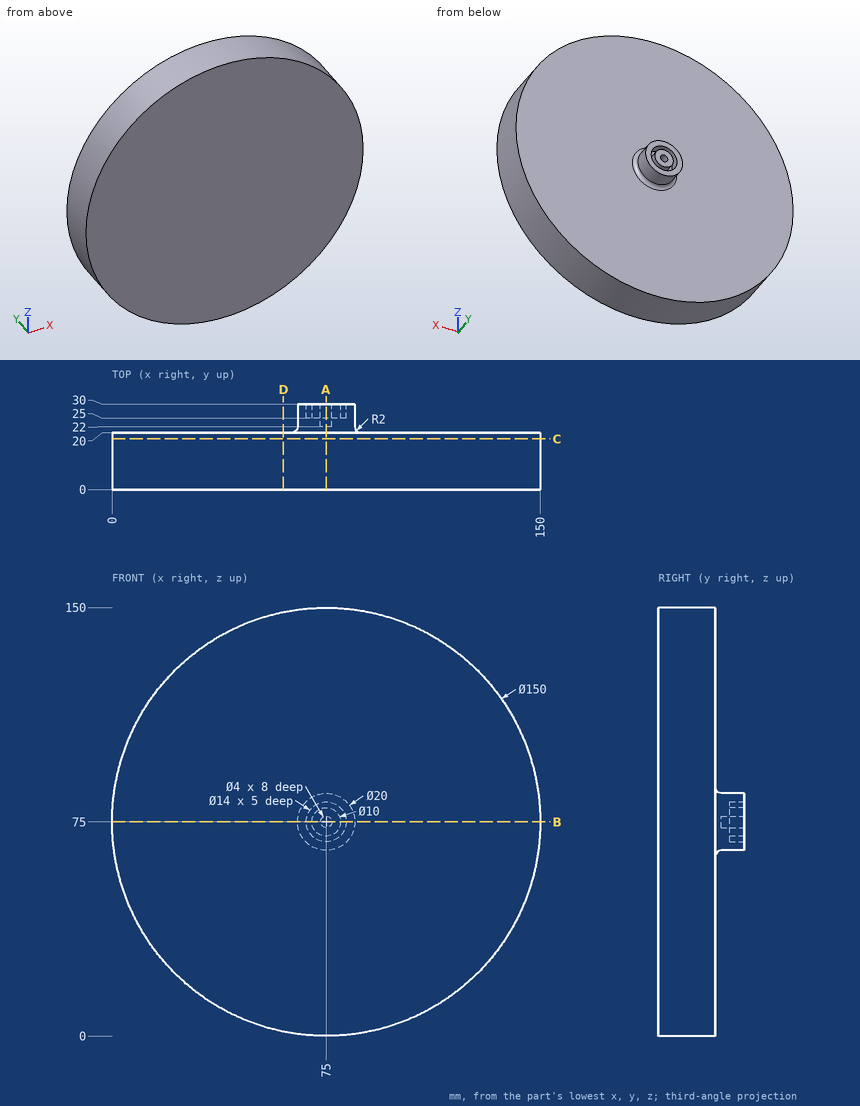
Design review of the part shown in the three views and the two pictorial views. Dimensions are in mm from the part's minimum x, y and z. Round coordinates to 2 decimals unless told otherwise and drop trailing zeros. Order: outer loops, then holes, each group sorted by start corner. A loop starts at its lowest first (then second) coordinate and runs counter-clockwise, first axis right, second up. Notation, with made-up numbers: (42.25, 13) -> (89.25, 13) arc R25 ccw to (89.25, 37) -> close; hole circle Ø10 at (-27, 51). An arc over 180 degrees is marked (long way). Write item = value, one per line. Start each with the question number.
1) To check wall thickness, follow line 1 (Z direction, x = 75, y = 28.55); line 2 (Z direction, x = 75, y = 24.5). State the ranges of each line that lie inside material, in increasing order. Write a range as from..to.
2) Insertion check: pin 1 (2 mm diameter, centred on y = 21.5, z = 93.5, fed in from -X); pin 2 (8 mm diameter, centred on y = 5, z = 48, fed in from +X); pin 3 (1.2 mm diameter, centred on x = 76, z = 75, fed in from +Y); pin 4 (5 mm diameter, centred on x = 26.5, y = 13.5, fed in from -Z). Each pin has a flat end and moves straight along its axis. Give the tip position at first contact, or say it passes through.
3) Take a section at A-A on x = 75. State the section outline as (y, z) points.
4) Take a section at B-B on z = 75. State the section outline as (x, y) points, plus the area to 3 significant figures.
5) Take a section at C-C on y = 17.75. State the section outline as (x, z) points.
6) Take a section at D-D on x = 60. State the section outline as (y, z) points, plus the area to 3 significant figures.
Verdict:
q1.line_1 = 65..68, 70..73, 77..80, 82..85
q1.line_2 = 65..73, 77..85
q2.pin_1 = through
q2.pin_2 = 146.39
q2.pin_3 = 22
q2.pin_4 = 15.76
q3.outline = (0, 0) -> (20, 0) -> (20, 63) arc R2 cw to (22, 65) -> (30, 65) -> (30, 68) -> (25, 68) -> (25, 70) -> (30, 70) -> (30, 73) -> (22, 73) -> (22, 77) -> (30, 77) -> (30, 80) -> (25, 80) -> (25, 82) -> (30, 82) -> (30, 85) -> (22, 85) arc R2 cw to (20, 87) -> (20, 150) -> (0, 150) -> close
q4.outline = (0, 0) -> (150, 0) -> (150, 20) -> (87, 20) arc R2 cw to (85, 22) -> (85, 30) -> (82, 30) -> (82, 25) -> (80, 25) -> (80, 30) -> (77, 30) -> (77, 22) -> (73, 22) -> (73, 30) -> (70, 30) -> (70, 25) -> (68, 25) -> (68, 30) -> (65, 30) -> (65, 22) arc R2 cw to (63, 20) -> (0, 20) -> close
q4.area = 3,150 mm2
q5.outline = circle Ø150 at (75, 75)
q6.outline = (0, 1.52) -> (20, 1.52) -> (20, 148.48) -> (0, 148.48) -> close
q6.area = 2,940 mm2
